```python
from build123d import *

# Parameters (mm, degrees)
F0_R            = 18.25
F0_R_2          = 16.25
F1_DEPTH        = 1800
F2_R            = 48.25
F2_R_2          = 18.25
F2_R_3          = 16.25
F3_DEPTH        = 5
F5_D            = 8.8
F5_COPIES_COUNT = 6


# Not quite as in the source:
# - a pattern or mirror of a feature is missing from the dataset's text; its kind, count and spacing are read off the source's solid


with BuildPart() as f1:
    # F0 (on Front) → F1 (new body)
    with BuildSketch(Plane.XZ):
        Circle(F0_R)
        Circle(F0_R_2, mode=Mode.SUBTRACT)
    extrude(amount=F1_DEPTH)

    # F2 (on face) → F3 (join)
    with BuildSketch(Plane.XZ.offset(1800)):
        Circle(F2_R)
        Circle(F2_R_2, mode=Mode.SUBTRACT)
        Circle(F2_R_2)
        Circle(F2_R_3, mode=Mode.SUBTRACT)
    extrude(amount=F3_DEPTH)

    # F5 (through all)
    with Locations(Plane.XZ.offset(1805)):
        with Locations((0, 31.25)):
            f5 = Hole(F5_D / 2)

    # F5_copies: F5 ×6 about axis
    f5_copies_axis = Axis((0, 0, 0), (0, 1, 0))
    for i in range(1, F5_COPIES_COUNT):
        add(f5.rotate(f5_copies_axis, i * 360 / F5_COPIES_COUNT), mode=Mode.SUBTRACT)


solid = f1.part
```
Geometry check sheet. Reference: the model listing, model coordinates, mm. A direction names the side the tool comes from. Coordinates: 2 decimals unless noted, no trailing zeros. Write each loop counter-clockwise with the first axis right and the second up, starting at its lowest first coordinate (ties: lowest second). Pieces come first, ordered by that corner, then holes. Notation, with made-up numbers: (24.25, 41.25) -> (38.25, 41.25) arc R34 cw to (38.25, 79.25) -> close; hole circle Ø7 at (-36.75, 17). An arc over 180 degrees is marked (long way). Use CSV: the item, a comma, the result in double quotes. Start each with the question number.
Item 1: Set-up check for faces 1 (the cylindrical face through (-48.203, -1802.465, 2.121)), 2 (the cylindrical face through (-3.956, -887.4, -17.816)): record each of +Z, -Z, +X, -X, +Y, -Y from which the full face is reachable in a straight line by a thin tool's end or side.
Item 2: Thickness scan on line 1 (X direction, y = -1639, z = -1.5); line 2 (X direction, y = -1152, z = 2.5); line 3 (Z direction, x = 0, y = -1052). Record the ranges inside material, lowest first.
Item 3: Cross-section at A-A, the plane y = -487. Record the cut outline in (x, z).
Item 4: Depth check by flat-ended pin: pin 1 Ø3 at (x, z) = (7, 26) entering from +Y; pin 2 Ø12 at (x, z) = (28, 19.5) entering from -Y. Enter the tip coordinate at first touch or a pass-through.
Answers:
1,face 1,"+Y, -Y"
1,face 2,"+Y"
2,line 1,"-18.19 to -16.18, 16.18 to 18.19"
2,line 2,"-18.08 to -16.06, 16.06 to 18.08"
2,line 3,"-18.25 to -16.25, 16.25 to 18.25"
3,outline,"circle Ø36.5 at (0, 0); hole circle Ø32.5 at (0, 0)"
4,pin 1,"y = -1800"
4,pin 2,"y = -1805"
